```python
from build123d import *

# Parameters (mm, degrees)
EXTRUDE_THIN1_DEPTH = 184.15
FILLET1_R           = 1.27


with BuildPart() as part:
    # Sketch1 → Extrude-Thin1 (new body)
    with BuildSketch(Plane.XY):
        with BuildLine():
            Line((0, 0), (-3.163716198, 0))
            Line((-3.163716198, 0), (-3.163716198, 2.119463738))
            ThreePointArc((-3.163716198, 2.119463738), (-3.923538192, 6.196525566), (-6.100987039, 9.72618265))
            ThreePointArc((-6.100987039, 9.72618265), (-6.193680003, 9.830012941), (-6.284653862, 9.935352736))
            ThreePointArc((-6.284653862, 9.935352736), (-6.972873445, 13.371716383), (-4.421808228, 15.774695279))
            Line((-4.421808228, 15.774695279), (-4.421808228, 18.25625))
            Line((-4.421808228, 18.25625), (0, 18.25625))
            Line((0, 18.25625), (0, 16.98625))
            Line((0, 16.98625), (-3.151808228, 16.98625))
            Line((-3.151808228, 16.98625), (-3.151808228, 14.585167393))
            ThreePointArc((-3.151808228, 14.585167393), (-5.570244387, 13.426967033), (-5.316692669, 10.757515207))
            ThreePointArc((-5.316692669, 10.757515207), (-5.239362872, 10.667974045), (-5.160571796, 10.579715995))
            ThreePointArc((-5.160571796, 10.579715995), (-2.738796161, 6.654003785), (-1.893716198, 2.119463738))
            Line((-1.893716198, 2.119463738), (-1.893716198, 1.27))
            Line((-1.893716198, 1.27), (0, 1.27))
            Line((0, 1.27), (0, 0))
        make_face()
    extrude(amount=-EXTRUDE_THIN1_DEPTH)

    # Fillet1
    fillet1_edges = [part.edges().sort_by_distance(p)[0] for p in [
        (-3.163716198, 0, -92.075),
        (-4.421808228, 18.25625, -92.075),
        (-3.151808228, 14.585167393, -92.075),
    ]]
    fillet(fillet1_edges, radius=FILLET1_R)


solid = part.part
```
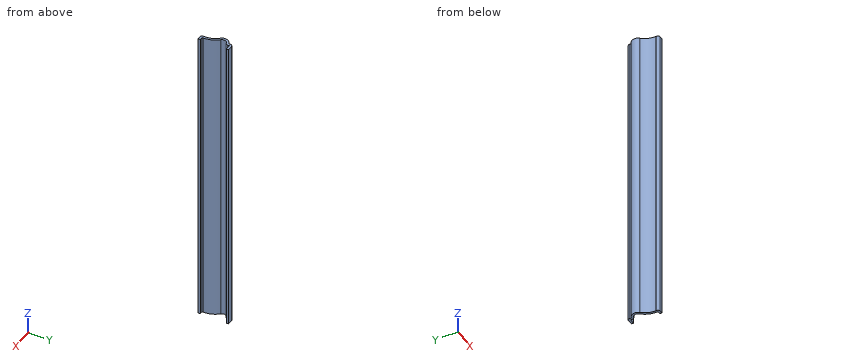
Design review of the part built by this model. Coordinates are the model's own, in mm. Give positions to 0.01 mm unless a question says otherwise; leave off trailing zeros. Write each loop counter-clockwise with the first axis right and the second up, starting at its lowest first coordinate (ties: lowest second). Pieces come first, ordered by that corner, then holes.
(1) Add section A-A (z = -169). Give the boundary of the cut face in (x, y), and give its area (3 significant figures).
Checked values:
outline: (-6.28, 9.94) arc R8.47 ccw to (-6.1, 9.73) arc R11.32 cw to (-3.16, 2.12) - (-3.16, 1.27) arc R1.27 ccw to (-1.89, 0) - (0, 0) - (0, 1.27) - (-1.89, 1.27) - (-1.89, 2.12) arc R12.59 ccw to (-5.16, 10.58) arc R7.2 cw to (-5.32, 10.76) arc R2.34 cw to (-4.11, 14.54) arc R1.27 ccw to (-3.15, 15.77) - (-3.15, 16.99) - (0, 16.99) - (0, 18.26) - (-3.15, 18.26) arc R1.27 ccw to (-4.42, 16.99) - (-4.42, 15.77) arc R3.61 ccw to start
area: 31.8 mm2
(2) Wall thickness on line 1 along Y through (x, z) = (-1.75, -70.5); line 2 along Y through (x, z) = (-4.25, -30.5); line 3 along X through (y, z) = (2.75, -72.5): over which ranges is each line inside the solid? List them lowest first.
Checked values:
line 1: y = 0 to 1.27, 16.99 to 18.26
line 2: y = 6.96 to 9.45, 14.5 to 17.62
line 3: x = -3.18 to -1.91
(3) Add section B-B (y = 4.75). Give the boundary of the cut face in (x, z), and give its area (3 significant figures).
Checked values:
outline: (-3.47, -184.15) - (-2.17, -184.15) - (-2.17, 0) - (-3.47, 0) - close
area: 240 mm2
(4) Clearance check with flat-ended pins moving along their axes: pin 1 Ø1 at (y, z) = (16.5, -105) entering from -X; pin 2 Ø0.7 at (y, z) = (1.5, -55) entering from -X; pin 3 Ø2.5 at (x, z) = (-2, -90) entering from -Y; pin 4 Ø0.6 at (y, z) = (16.5, -137) entering from +X. State where each tip first meets the part, or that it passes through.
Checked values:
pin 1: stops at x = -4.42
pin 2: stops at x = -3.16
pin 3: stops at y = 0
pin 4: stops at x = -3.15
